```python
from build123d import *

# Parameters (mm, degrees)
F0_R     = 11
F0_R_2   = 9
F1_DEPTH = 3.5
F0_R_3   = 6
F0_R_4   = 4
F2_DEPTH = 3
F3_SIZE  = 0.3


with BuildPart() as f1:
    # F0 (on Top) → F1 (new body, symmetric)
    with BuildSketch(Plane.XY):
        Circle(F0_R)
        Circle(F0_R_2, mode=Mode.SUBTRACT)
    extrude(amount=F1_DEPTH, both=True)



with BuildPart() as f1b:
    # F0 (on Top) → F1, piece 2 (new body, symmetric)
    with BuildSketch(Plane.XY):
        Circle(F0_R_3)
        Circle(F0_R_4, mode=Mode.SUBTRACT)
    extrude(amount=F1_DEPTH, both=True)


with BuildPart() as f1_1:
    add(f1.part)

    add(f1b.part)  # F2 merges F1b
    # F0 (on Top) → F2 (join, symmetric)
    with BuildSketch(Plane.XY):
        Circle(F0_R_2)
        Circle(F0_R_3, mode=Mode.SUBTRACT)
    extrude(amount=F2_DEPTH, both=True)

    # F3
    f3_edges = [f1_1.edges().sort_by_distance(p)[0] for p in [
        (-11, 0, 3.5),
        (-4, 0, 3.5),
        (-9, 0, 3.5),
        (-6, 0, 3.5),
        (-11, 0, -3.5),
        (-9, 0, -3.5),
        (-6, 0, -3.5),
        (-4, 0, -3.5),
    ]]
    chamfer(f3_edges, length=F3_SIZE)


solid = f1_1.part
```
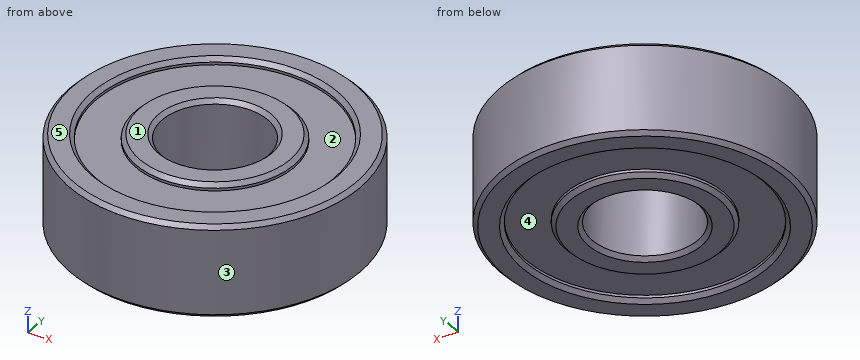
Source: CAD feature listing. Evaluate the final solid. Frame: model axes, mm. Face numbers are marked on the shaded views. A direction names the side the tool comes from. Round coordinates to 2 decimals unless told otherwise and drop trailing zeros. Loops run counter-clockwise (first coordinate to the right, second up) from the corner with the lowest first, then second, coordinate; pieces in that order, holes last.
1. Section query A-A on z = 1.5. Output: boundary loops of the cut face in (x, y), and give its area (3 significant figures).
2. Mould query, pull axis X, two halves, no side actions, for the marked faces 3, 4 and 5. Classes: released by +X, released by -X, zero draft, split by the parting line, or undercut.
3. Contact query for flat-ended pins moving along their axis: pin 1 (2 mm diameter, centred on y = 3.5, z = -1, fed in from -X); pin 2 (3 mm diameter, centred on x = -4, z = 2, fed in from -Y); pin 3 (1 mm diameter, centred on y = 6, z = 0, fed in from +X). Output: stop coordinate, or through.
4. Ray query, L1, parallel to Y at x = 0, z = 3.05; L2, parallel to Y at x = -1.5, z = 3.25; L3, parallel to Y at x = 0, z = -0.5. Return the intervals inside material, ascending.
5. Access query for the marked faces 1 and 2. Directions: +Z, -Z, +X, -X, +Y, -Y. A direction counts if a zero-diameter tool reaches every point of the face in a straight line with its end or side. Return the directions, or none.
Answers below:
1. outline: circle Ø22 at (0, 0); hole circle Ø8 at (0, 0)
1. area: 330 mm2
2. face 3: split by the parting line
2. face 4: undercut
2. face 5: zero draft
3. pin 1: stops at x = -10.71
3. pin 2: stops at y = -10.71
3. pin 3: stops at x = 9.53
4. L1: y = -11 to -9, -6 to -4, 4 to 6, 9 to 11
4. L2: y = -10.85 to -8.92, -5.76 to -3.76, 3.76 to 5.76, 8.92 to 10.85
4. L3: y = -11 to -4, 4 to 11
5. face 1: +Z, +X, -X, +Y, -Y
5. face 2: +Z
